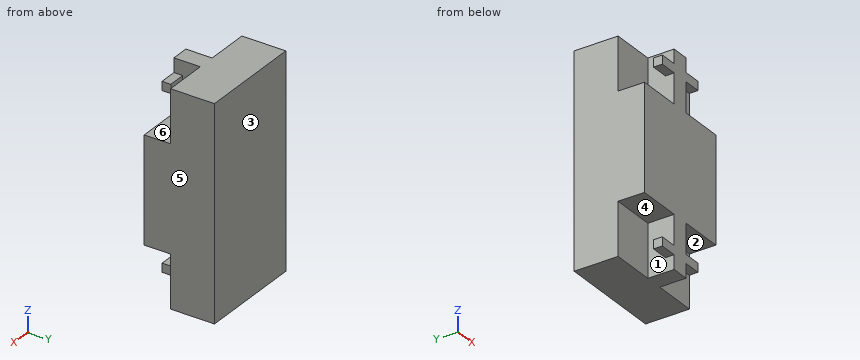
from build123d import *

# Parameters (mm, degrees)
BOSS_EXTRUDE1_DEPTH      = 150
BOSS_EXTRUDE1_DEPTH_BACK = 150
SKETCH2_W                = 600
SKETCH2_H                = 200
SKETCH3_W                = 150
SKETCH3_H                = 75
CUT_EXTRUDE1_DEPTH       = 125
SKETCH4_W                = 25
SKETCH4_H                = 25
BOSS_EXTRUDE2_DEPTH      = 50
MIRROR3_COPY_1_SKETCH_W  = 25
MIRROR3_COPY_1_SKETCH_H  = 25
MIRROR3_COPY_1_DEPTH     = 50


with BuildPart() as part:
    # Sketch2 → Boss-Extrude1 (new, two sides: drawn at the far end of the back side and taken through both)
    with BuildSketch(Plane(origin=(0, 0, 0), x_dir=(0, 0, -1), z_dir=(1, 0, 0)).offset(-BOSS_EXTRUDE1_DEPTH_BACK)):
        Rectangle(SKETCH2_W, SKETCH2_H)
    extrude(amount=BOSS_EXTRUDE1_DEPTH + BOSS_EXTRUDE1_DEPTH_BACK)

    # Sketch3 → Cut-Extrude1 (cut)
    with BuildSketch(Plane(origin=(150, 0, 0), x_dir=(0, 0, -1), z_dir=(1, 0, 0))):
        with Locations((-225, -62.5)):
            Rectangle(SKETCH3_W, SKETCH3_H)
        with Locations((225, -62.5)):
            Rectangle(SKETCH3_W, SKETCH3_H)
    cut_extrude1 = extrude(amount=-CUT_EXTRUDE1_DEPTH, mode=Mode.SUBTRACT)

    # Mirror1: Cut-Extrude1 across plane
    add(cut_extrude1.mirror(Plane(origin=(0, 0, 0), x_dir=(0, 0, 1), z_dir=(1, 0, 0))), mode=Mode.SUBTRACT)

    # Sketch4 → Boss-Extrude2 (add)
    with BuildSketch(Plane(origin=(25, 0, 0), x_dir=(0, 0, -1), z_dir=(1, 0, 0))):
        with Locations((-247.5, -87.5)):
            Rectangle(SKETCH4_W, SKETCH4_H)
    boss_extrude2 = extrude(amount=BOSS_EXTRUDE2_DEPTH)

    # Mirror2: Boss-Extrude2 across plane
    add(boss_extrude2.mirror(Plane(origin=(0, 0, 0), x_dir=(0, 0, 1), z_dir=(1, 0, 0))))

    # Mirror3: Boss-Extrude2 across plane
    add(boss_extrude2.mirror(Plane.XY))

    # Mirror3 copy 1 sketch → Mirror3 copy 1 (add)
    with BuildSketch(Plane.ZY.offset(25)):
        with Locations((-247.5, -87.5)):
            Rectangle(MIRROR3_COPY_1_SKETCH_W, MIRROR3_COPY_1_SKETCH_H)
    extrude(amount=MIRROR3_COPY_1_DEPTH)


solid = part.part
The listing builds one solid part. Answer for the finished solid, in the listing's coordinates (mm). Face numbers are marked on the shaded views. A direction names the side the tool comes from. Round coordinates to 2 decimals unless told otherwise and drop trailing zeros. Order: outer loops, then holes, each group sorted by start corner. A loop starts at its lowest first (then second) coordinate and runs counter-clockwise, first axis right, second up. Notation, with made-up numbers: (18, 87.25) - (24, 87.25) arc R25 cw to (24, 115.25) - close; hole circle Ø6 at (-11, -29.5). An arc over 180 degrees is marked (long way). Write item = value, one per line. Start each with the question number.
1) Section D-D, the plane x = 89 is taken. Write down the section's boundary in (y, z).
2) Section B-B, the plane z = -216.5 is taken. Write down the section's boundary in (x, y).
3) Straight lines are drawn through the part: L1, parallel to Z at x = 63, y = -85.5; L2, parallel to Y at x = 48, z = 236; L3, parallel to X at y = -67, z = -163. For each, find the intervals that lie inside material, in ascending order.
4) For a pull along Y with two mould halves and no side action, classify the marked faces 1, 2 and 3 as released by +Y, released by -Y, zero draft, split by the parting line, or undercut.
5) Section C-C, the plane y = -42.5 is taken. Write down the section's boundary in (x, z), plus the area to 3 significant figures.
6) Given pin 1 (22.5 mm diameter, centred on x = 83, y = -59, fed in from -Z); pin 2 (12.5 mm diameter, centred on y = -93.5, z = 242, fed in from -X); pin 3 (3 mm diameter, centred on x = 60, z = -227.5, fed in from -Y), each flat-ended and moving along its own axis, determine where each tip first touches the part or whether it passes through.
7) For the marked faces 4, 5 and 6, determine the directions among +Z, -Z, +X, -X, +Y, -Y from which every point of the face is accessible in a straight line to the end or side of a thin tool.
8) Section A-A, the plane x = 35 is taken. Write down the section's boundary in (y, z).
Results list:
q1.outline = (-100, -150) - (-25, -150) - (-25, -300) - (100, -300) - (100, 300) - (-25, 300) - (-25, 150) - (-100, 150) - close
q2.outline = (-150, -25) - (-25, -25) - (-25, -100) - (25, -100) - (25, -25) - (150, -25) - (150, 100) - (-150, 100) - close
q3.L1 = -260 to -235, -150 to 150, 235 to 260
q3.L2 = -100 to -75, -25 to 100
q3.L3 = -25 to 25
q4.face_1 = undercut
q4.face_2 = zero draft
q4.face_3 = released by +Y
q5.outline = (-150, -150) - (-25, -150) - (-25, -300) - (25, -300) - (25, -150) - (150, -150) - (150, 150) - (25, 150) - (25, 300) - (-25, 300) - (-25, 150) - (-150, 150) - close
q5.area = 105,000 mm^2
q6.pin_1 = -150
q6.pin_2 = -75
q6.pin_3 = -25
q7.face_4 = -X, -Y
q7.face_5 = +Z, -Z, +X, +Y, -Y
q7.face_6 = +X, -Y
q8.outline = (-100, -260) - (-75, -260) - (-75, -235) - (-100, -235) - close; (-100, -150) - (-25, -150) - (-25, -300) - (100, -300) - (100, 300) - (-25, 300) - (-25, 150) - (-100, 150) - close; (-100, 235) - (-75, 235) - (-75, 260) - (-100, 260) - close
